```python
from build123d import *

# Parameters (mm, degrees)
BOSS_EXTRUDE1_DEPTH      = 6
BOSS_EXTRUDE1_DEPTH_BACK = 6
CHAMFER1_SIZE            = 0.2


with BuildPart() as part:
    # Sketch3 → Boss-Extrude1 (new, two sides: drawn at the far end of the back side and taken through both)
    with BuildSketch(Plane.XY.offset(-BOSS_EXTRUDE1_DEPTH_BACK)):
        with BuildLine():
            Line((-35, 12.5), (0, 12.5))
            Line((0, 12.5), (0, -12.5))
            Line((0, -12.5), (-35, -12.5))
            Line((-35, -12.5), (-35, 0.5))
            Line((-35, 0.5), (-21.898979486, 0.5))
            ThreePointArc((-21.898979486, 0.5), (-12, 1.5), (-21.898979486, 2.5))
            Line((-21.898979486, 2.5), (-35, 2.5))
            Line((-35, 2.5), (-35, 12.5))
        make_face()
    extrude(amount=BOSS_EXTRUDE1_DEPTH + BOSS_EXTRUDE1_DEPTH_BACK)

    # Sketch5 → Cut-Revolve1 (revolve, cut)
    with BuildSketch(Plane.XY):
        Polygon((-32.5, 12.5), (-32.5, 5.5), (-30.25, 5.5), (-30.25, -12.5), (-27.5, -12.5), (-27.5, 1.5), (-27.5, 5.5), (-27.5, 12.5), align=None)
    revolve(axis=Axis((-27.5, 12.5, 0), (0, -1, 0)), mode=Mode.SUBTRACT)

    # Chamfer1
    chamfer1_edges = [part.edges().sort_by_distance(p)[0] for p in [
        (-12, 1.5, 6),
        (-28.449489743, 0.5, 6),
        (-28.449489743, 0.5, -6),
        (-12, 1.5, -6),
        (-28.449489743, 2.5, -6),
        (-24.75, -12.5, 0),
        (-22.5, 12.5, 0),
        (-28.449489743, 2.5, 6),
    ]]
    chamfer(chamfer1_edges, length=CHAMFER1_SIZE)

    # Mirror1: part across plane


with BuildPart() as part_1:
    add(part.part)
    add(part.part.mirror(Plane(origin=(0, 0, 0), x_dir=(0, 0, 1), z_dir=(1, 0, 0))))


solid = part_1.part
```
Can you work these out from the model? Positions are in its coordinate system, mm. A direction names the side the tool comes from. Coordinates: 2 decimals unless noted, no trailing zeros. Write each loop counter-clockwise with the first axis right and the second up, starting at its lowest first coordinate (ties: lowest second). Pieces come first, ordered by that corner, then holes. Notation, with made-up numbers: (85, 66) - (98, 66) arc R28 cw to (98, 96) - close; hole circle Ø3 at (-37, -37.5). An arc over 180 degrees is marked (long way). Return JSON: item names as keys, results as strings.
Q1. I'm going to push a flat-ended pin straight in: pin 1 Ø3.5 at (x, z) = (29.5, 1.5) entering from +Y. Where does the tip first touch, or does it pass through?
Computed values:
{"pin 1": "stops at y = 5.5"}
Q2. Thinking about a two-plate mould opening in Y: for faces 1 (the cylindrical face through (-24.753, 3.979, -0.121)), 2 (the flat face through (0, 12.5, 0)), 3 (the flat face through (-29, 0.5, -3)), which applies, +Y half, -Y half, draft (parallel to the pull), parting line (faces both ways), or undercut?
Computed values:
{"face 1": "draft", "face 2": "+Y half", "face 3": "undercut"}
Q3. Please list where these lines run through material, in increasing order: L1, parallel to X at y = -4.5, z = 0; L2, parallel to Z at x = 27.5, y = -7; L3, parallel to Z at x = 27.5, y = 7. Write a range as from..to.
Computed values:
{"L1": "x = -35..-30.25, -24.75..24.75, 30.25..35", "L2": "z = -6..-2.75, 2.75..6", "L3": "z = -6..-5, 5..6"}
Q4. If we section it at B-B (x = -17): Please give me the cut outline in (y, z).
Computed values:
{"outline": "(-12.5, -6) - (-3.7, -6) - (-3.5, -5.8) - (-3.5, 5.8) - (-3.7, 6) - (-12.5, 6) - close; (6.5, -5.8) - (6.7, -6) - (12.5, -6) - (12.5, 6) - (6.7, 6) - (6.5, 5.8) - close"}
Q5. If we section it at D-D (y = 1.5): Please give me the cut outline in (x, z).
Computed values:
{"outline": "(-12, -5.8) - (-11.8, -6) - (11.8, -6) - (12, -5.8) - (12, 5.8) - (11.8, 6) - (-11.8, 6) - (-12, 5.8) - close"}
Q6. If we section it at C-C (y = -6.75): Please give me the cut outline in (x, z).
Computed values:
{"outline": "(-35, -6) - (35, -6) - (35, 6) - (-35, 6) - close; hole circle Ø5.5 at (-27.5, 0); hole circle Ø5.5 at (27.5, 0)"}
Q7. On a 3-axis mill with a long thin cutter (end or side, diameter ignored), from which of +Z, -Z, +X, -X, +Y, -Y can I reach the whole of each face in a straight line? I mean faces 4 (the flat face through (-28, 2.5, -3)), 5 (the cylindrical face through (-24.753, -5.99, -0.121)), 6 (the flat face through (28, 2.5, -3)). Say none if no direction works.
Computed values:
{"face 4": "+Z, -Z, -X", "face 5": "+Y, -Y", "face 6": "+Z, -Z, +X"}
Q8. If we section it at A-A (x = -27.5): Please give me the cut outline in (y, z).
Computed values:
{"outline": "(-12.5, -6) - (0.3, -6) - (0.5, -5.8) - (0.5, -2.75) - (-12.3, -2.75) - (-12.5, -2.95) - close; (-12.5, 2.95) - (-12.3, 2.75) - (0.5, 2.75) - (0.5, 5.8) - (0.3, 6) - (-12.5, 6) - close; (2.5, -5.8) - (2.7, -6) - (12.5, -6) - (12.5, -5.2) - (12.3, -5) - (5.5, -5) - (5.5, -2.75) - (2.5, -2.75) - close; (2.5, 2.75) - (5.5, 2.75) - (5.5, 5) - (12.3, 5) - (12.5, 5.2) - (12.5, 6) - (2.7, 6) - (2.5, 5.8) - close"}
